Autodesk Fusion 360 part; units mm, degrees
sketch "Sketch1" plane through (0, 0, 0) normal (0, 0, 1) x (1, 0, 0)
  line L0 (50, 30) -> (110, 30)
  line L1 (110, 30) -> (110, 50)
  line L2 (110, 50) -> (50, 50)
  line L3 (50, 50) -> (50, 30)
  line L4 (110, 30) -> (60, 30)
  line L5 (60, 30) -> (60, 40)
  line L6 (60, 40) -> (110, 40)
  line L7 (110, 40) -> (110, 30)
  line L8 (50, 50) -> (70, 50)
  line L9 (70, 50) -> (70, -10)
  line L10 (70, -10) -> (50, -10)
  line L11 (50, -10) -> (50, 50)
  line L12 (60, 40) -> (70, 40)
  line L13 (70, 40) -> (70, -10)
  line L14 (70, -10) -> (60, -10)
  line L15 (60, -10) -> (60, 40)
  dimension "d1" = 60
  dimension "d2" = 20
  dimension "d3" = 50
  dimension "d4" = 10
  dimension "d5" = 20
  dimension "d6" = 60
extrude "Extrude1" add sketch "Sketch1" along normal blind 4 contours L0 L2 L3 L5 L6 L8 L9 L11 L12 L15 | L0 L10 L11 L15 | L1 L2 L6 L9
extrude "Extrude2" add sketch "Sketch1" along normal blind 64 contours L0 L4 L5 L6 L9 L12 L13 L15 | L0 L4 L9 L10 L13 L14 L15 | L0 L1 L4 L6 L7 L9 L13
sketch "Sketch2" plane through (0, 0, 64) normal (0, 0, 1) x (-1, 0, 0)
  line L0 (-60, 10) -> (-70, 10)
  line L1 (-70, 10) -> (-70, -30)
  line L2 (-70, -30) -> (-110, -30)
  line L3 (-110, -30) -> (-110, -40)
  line L4 (-110, -40) -> (-60, -40)
  line L5 (-60, -40) -> (-60, 10)
  line L6 (-70, 10) -> (-50, 10)
  line L7 (-50, 10) -> (-50, -50)
  line L8 (-50, -50) -> (-70, -50)
  line L9 (-70, -50) -> (-70, 10)
  line L10 (-70, -30) -> (-110, -30)
  line L11 (-110, -30) -> (-110, -50)
  line L12 (-110, -50) -> (-70, -50)
  line L13 (-70, -50) -> (-70, -30)
extrude "Extrude3" add sketch "Sketch2" along normal blind 4
sketch "Sketch3" plane through (0, 0, 68) normal (0, 0, 1) x (-1, 0, 0)
  line L0 (-70, -30) -> (-110, -30)
  line L1 (-110, -30) -> (-110, -50)
  line L2 (-110, -50) -> (-50, -50)
  line L3 (-50, -50) -> (-50, 10)
  line L4 (-50, 10) -> (-70, 10)
  line L5 (-70, 10) -> (-70, -30)
  line L6 (-75, -25) -> (-65, -25)
  line L7 (-65, -25) -> (-65, -35)
  line L8 (-65, -35) -> (-75, -35)
  line L9 (-75, -35) -> (-75, -25)
extrude "Extrude4" cut sketch "Sketch3" against normal blind 68 contours L0 L5 L6 L7 L8 L9
fillet "Fillet1" radius 4 2 edges at (80, 50, 4) (50, 20, 4)
fillet "Fillet2" radius 4 2 edges at (80, 50, 64) (50, 20, 64)
fillet "Fillet3" radius 2 1 edges at (110, 40, 34)
fillet "Fillet4" radius 2 1 edges at (60, -10, 34)
fillet "Fillet5" radius 2 1 edges at (60, 40, 34)
Model file for the job. Use its own axes, mm. A direction names the side the tool comes from. Round coordinates to 2 decimals unless told otherwise and drop trailing zeros. Order: outer loops, then holes, each group sorted by start corner. A loop starts at its lowest first (then second) coordinate and runs counter-clockwise, first axis right, second up. Notation, with made-up numbers: (43, -13.75) -> (70, -13.75) arc R6 cw to (70, -6.75) -> close; hole circle Ø3 at (77, 34.25). An arc over 180 degrees is marked (long way). Use one line per item in the form item = value.
Item 1: Flat gauge pins, fed straight in: pin 1 Ø10.5 at (x, z) = (100, 44) entering from -Y; pin 2 Ø1 at (y, z) = (10.5, 60) entering from -X; pin 3 Ø14 at (x, z) = (84.5, 36) entering from +Y. Where does each tip first touch, or does it go through?
Returned:
pin_1 = 30
pin_2 = 60
pin_3 = 40
Item 2: Tool access for faces 5 (the face through (60.6, 39.43, 34.42)), 6 (the face through (75, 33, 34)), 7 (the face through (60, 15, 34)), 8 (the face through (85, 40, 34)): list every direction of +Z, -Z, +X, -X, +Y, -Y with a clear straight run to the whole face (end or side of a thin tool).
Returned:
face_5 = -X, +Y
face_6 = +Z, -Z, -Y
face_7 = -X, +Y, -Y
face_8 = +X, -X, +Y
Item 3: Cut at D-D, the plane z = 58.5. Write the cut outline in (x, y), and give its area (3 significant figures).
Returned:
outline = (60, -8) arc R2 ccw to (62, -10) -> (70, -10) -> (70, 25) -> (65, 25) -> (65, 35) -> (75, 35) -> (75, 30) -> (110, 30) -> (110, 38) arc R2 ccw to (108, 40) -> (62, 40) arc R2 ccw to (60, 38) -> close
area = 822 mm^2
Item 4: Drill centre lines: line 1 (X direction, y = 31, z = 37); line 2 (Z direction, x = 96, y = 41.5); line 3 (X direction, y = -6, z = 58). Where is each one in solid material? Low to high.
Returned:
line_1 = 60 to 65, 75 to 110
line_2 = 0 to 4, 64 to 68
line_3 = 60 to 70
Item 5: Pull direction Y, two halves, no side cores. Call faces 1 (the face through (60.57, -9.4, 34.42)), 2 (the face through (80.42, 48.797, 65.14)), 3 (the face through (80, 33, 68)), 4 (the face through (68, 25, 34)): released by +Y, released by -Y, zero draft, split by the parting line, or undercut.
Returned:
face_1 = released by -Y
face_2 = released by +Y
face_3 = zero draft
face_4 = undercut
